from build123d import *

# Parameters (mm, degrees)
SKETCH1_W                       = 19.05
SKETCH1_H                       = 101.6
BOSS_EXTRUDE1_DEPTH             = 9.525
SKETCH2_W                       = 6.35
SKETCH2_H                       = 9.525
CUT_EXTRUDE1_DEPTH              = 103.489078686
F_1_4_0_25_DIAMETER_HOLE1_D     = 6.35
F_1_4_0_25_DIAMETER_HOLE1_DEPTH = 25.4
F_1_4_0_25_DIAMETER_HOLE1_TIP   = 1.907732465
FILLET1_R                       = 12.7
FILLET2_R                       = 6.35


with BuildPart() as part:
    # Sketch1 → Boss-Extrude1 (new, symmetric)
    with BuildSketch(Plane(origin=(0, 0, 0), x_dir=(1, 0, 0), z_dir=(0, 1, 0))):
        Rectangle(SKETCH1_W, SKETCH1_H)
    extrude(amount=BOSS_EXTRUDE1_DEPTH, both=True)

    # Sketch2 → Cut-Extrude1 (cut, through all)
    with BuildSketch(Plane.XY.offset(50.8)):
        with Locations((6.35, -4.7625)):
            Rectangle(SKETCH2_W, SKETCH2_H)
    extrude(amount=-CUT_EXTRUDE1_DEPTH, mode=Mode.SUBTRACT)

    # 1/4 (0.25) Diameter Hole1
    with Locations(Plane(origin=(0, 9.525, 0), x_dir=(1, 0, 0), z_dir=(0, 1, 0))):
        with Locations((-3.175, 19.05), (-3.175, -19.05)):
            Hole(F_1_4_0_25_DIAMETER_HOLE1_D / 2, depth=F_1_4_0_25_DIAMETER_HOLE1_DEPTH)
            with Locations((0, 0, -(F_1_4_0_25_DIAMETER_HOLE1_DEPTH + F_1_4_0_25_DIAMETER_HOLE1_TIP / 2))):  # 118° drill point
                Cone(0, F_1_4_0_25_DIAMETER_HOLE1_D / 2, F_1_4_0_25_DIAMETER_HOLE1_TIP, mode=Mode.SUBTRACT)

    # Fillet1
    fillet1_edges = [part.edges().sort_by_distance(p)[0] for p in [
        (3.175, -4.7625, -50.8),
        (3.175, -4.7625, 50.8),
    ]]
    fillet(fillet1_edges, radius=FILLET1_R - 0.0001)  # a hair under: the kernel refuses the full size

    # Fillet2
    fillet2_edges = [part.edges().sort_by_distance(p)[0] for p in [
        (9.525, 4.7625, -50.8),
        (9.525, 4.7625, 50.8),
    ]]
    fillet(fillet2_edges, radius=FILLET2_R)


solid = part.part
Verification items for the finished model (mm, model axes). A direction names the side the tool comes from. Coordinates: 2 decimals unless noted, no trailing zeros. Order: outer loops, then holes, each group sorted by start corner. A loop starts at its lowest first (then second) coordinate and runs counter-clockwise, first axis right, second up. Notation, with made-up numbers: M -31.5,72.5 L 1.5,72.5 A33 cw 1.5,100.5 Z; hole C 22.5,61.25 d7. An arc over 180 degrees is marked long. Return JSON: item names as keys, results as strings.
1) Cross-section at C-C, the plane x = -4.25. Record the boundary of the cut face in (y, z) (3 decimals), and give its area (3 significant figures).
Answer list:
{"outline": "M -9.525,-49.653 L 0,-49.653 L 0,-50.8 L 9.525,-50.8 L 9.525,-22.037 L -9.525,-22.037 Z; M -9.525,-16.063 L 9.525,-16.063 L 9.525,16.063 L -9.525,16.063 Z; M -9.525,22.037 L 9.525,22.037 L 9.525,50.8 L 0,50.8 L 0,49.653 L -9.525,49.653 Z", "area": "1,690 mm2"}
2) Access from +Z, -Z, +X, -X, +Y, -Y to the whole of each face (thin tool, end or side, straight path). Record for faces 4 (the flat face through (3.175, -5, 1)), 5 (the cylindrical face through (-0.644, -4.696, -47.178)), 6 (the flat face through (-3, -9.525, -1)).
Answer list:
{"face 4": "+Z, -Z, +X, -Y", "face 5": "-Z, +X, -Y", "face 6": "+Z, -Z, +X, -X, -Y"}
3) Cross-section at D-D, the plane z = -6. Record the boundary of the cut face in (x, y) (3 decimals), and give its area (3 significant figures).
Answer list:
{"outline": "M -9.525,-9.525 L 3.175,-9.525 L 3.175,0 L 9.525,0 L 9.525,9.525 L -9.525,9.525 Z", "area": "302 mm2"}
4) Gauge pin test, flat ends, axial feed: pin 1 (1 mm diameter, centred on x = 6, z = 3.5, fed in from -Y); pin 2 (7.5 mm diameter, centred on x = -3.175, z = 19.05, fed in from -Y) (3 decimals); pin 3 (5 mm diameter, centred on y = -3, z = 0.5, fed in from +X) (3 decimals); pin 4 (4 mm diameter, centred on x = -3.175, z = -19.05, fed in from +Y). Record the tip position at first contact, or that the pin passes through.
Answer list:
{"pin 1": "y = 0", "pin 2": "y = -9.525", "pin 3": "x = 3.175", "pin 4": "through"}
5) Release check for a two-part mould opening along Z. For faces 1 (the cylindrical face through (-0.644, -4.696, 47.178)), 2 (the cylindrical face through (-2.49, -0.13, -15.95)), 3 (the flat face through (0, 9.525, -1)) record: +Z half, -Z half, draft (parallel to the pull), parting line (faces both ways), or undercut.
Answer list:
{"face 1": "+Z half", "face 2": "undercut", "face 3": "draft"}
6) Cross-section at A-A, the plane z = 19.05. Record the boundary of the cut face in (x, y) (3 decimals), and give its area (3 significant figures).
Answer list:
{"outline": "M -9.525,-9.525 L -6.35,-9.525 L -6.35,9.525 L -9.525,9.525 Z; M 0,-9.525 L 3.175,-9.525 L 3.175,0 L 9.525,0 L 9.525,9.525 L 0,9.525 Z", "area": "181 mm2"}
7) Thickness scan on L1, parallel to X at y = 5.25, z = -19.05 (3 decimals); L2, parallel to X at y = -2.75, z = -19.05 (3 decimals); L3, parallel to Z at x = -1.25, y = -2. Record the ranges inside material, lowest first. Write a range as [from, to].
Answer list:
{"L1": "[-9.525, -6.35], [0, 9.525]", "L2": "[-9.525, -6.35], [0, 3.175]", "L3": "[-47.73, -21.57], [-16.53, 16.53], [21.57, 47.73]"}
8) Cross-section at B-B, the plane y = 6. Record the boundary of the cut face in (x, z) (3 decimals), and give its area (3 significant figures).
Answer list:
{"outline": "M -9.525,-50.8 L 3.175,-50.8 A6.35 ccw 9.525,-44.45 L 9.525,44.45 A6.35 ccw 3.175,50.8 L -9.525,50.8 Z; hole C -3.175,-19.05 d6.35; hole C -3.175,19.05 d6.35", "area": "1,850 mm2"}
